Could you check a few things on this model? Use its own coordinates, in mm. A direction names the side the tool comes from. Coordinates: 2 decimals unless noted, no trailing zeros. Loops run counter-clockwise (first coordinate to the right, second up) from the corner with the lowest first, then second, coordinate; pieces in that order, holes last. Notation, with made-up numbers: (-7.75, -32) -> (50.25, -32) arc R27 ccw to (50.25, -13) -> close; hole circle Ø7 at (3, 16.25). An arc over 180 degrees is marked (long way). One line per question, with ' | ' between items.
```python
from build123d import *

# Parameters (mm, degrees)
SKETCH1_W                                            = 90
SKETCH1_H                                            = 30
BOSS_EXTRUDE1_DEPTH                                  = 3
SKETCH3_W                                            = 30
SKETCH3_H                                            = 3
BOSS_EXTRUDE2_DEPTH                                  = 60
RIB5_REACH                                           = 80.861
SKETCH8_WALL_W                                       = 225.516409736
SKETCH8_WALL_H                                       = 30
CUT_EXTRUDE2_REACH                                   = 85.03
SKETCH10_R                                           = 1.1
SKETCH12_R                                           = 2.5
CUT_EXTRUDE3_DEPTH                                   = 27
FILLET1_R                                            = 3
CUT_EXTRUDE4_REACH                                   = 85.03
FILLET2_R                                            = 2
CSK_FOR_M2_5_COUNTERSUNK_FLAT_HEAD_SCREW_D           = 2.7
CSK_FOR_M2_5_COUNTERSUNK_FLAT_HEAD_SCREW_CSINK_D     = 5.5
CSK_FOR_M2_5_COUNTERSUNK_FLAT_HEAD_SCREW_CSINK_ANGLE = 90
MIRROR1_AT_THE_SECOND_PLANE_COPY_1_D                 = 2.7
MIRROR1_AT_THE_SECOND_PLANE_COPY_1_CSINK_D           = 5.5
MIRROR1_AT_THE_SECOND_PLANE_COPY_1_CSINK_ANGLE       = 90


with BuildPart() as part:
    # Sketch1 → Boss-Extrude1 (new body)
    with BuildSketch(Plane(origin=(0, 0, 0), x_dir=(1, 0, 0), z_dir=(0, 1, 0))):
        Rectangle(SKETCH1_W, SKETCH1_H)
    extrude(amount=BOSS_EXTRUDE1_DEPTH)

    # Sketch3 → Boss-Extrude2 (add)
    with BuildSketch(Plane(origin=(0, 3, 0), x_dir=(1, 0, 0), z_dir=(0, 1, 0))):
        with Locations((0, -13.5)):
            Rectangle(SKETCH3_W, SKETCH3_H)
    extrude(amount=BOSS_EXTRUDE2_DEPTH)

    # Sketch8 wall → Rib5 (add, up to next)
    with BuildSketch(Plane(origin=(0, 33, -1.5), x_dir=(0, -0.911921505175, -0.410364677329), z_dir=(0, 0.410364677329, -0.911921505175)), mode=Mode.PRIVATE) as rib5_sk1:
        Rectangle(SKETCH8_WALL_W, SKETCH8_WALL_H)
    rib5_tool1 = extrude(rib5_sk1.sketch, amount=-RIB5_REACH, mode=Mode.PRIVATE) - part.part
    add(rib5_tool1.solids().sort_by_distance((0, 33, -1.5))[0])

    # Cut-Extrude2: up to this plane
    cut_extrude2_end = Plane(origin=(0, 63, 12), z_dir=(0, -0.410364677328798, 0.9119215051751063))
    # Sketch10 → Cut-Extrude2 (cut, up to the surface)
    with BuildSketch(Plane.XY.offset(15), mode=Mode.PRIVATE) as cut_extrude2_sk1:
        with Locations((-10, 56.3)):
            Circle(SKETCH10_R)
    cut_extrude2_tool1 = split(extrude(cut_extrude2_sk1.sketch, amount=-CUT_EXTRUDE2_REACH, mode=Mode.PRIVATE), bisect_by=cut_extrude2_end, keep=Keep.BOTH, mode=Mode.PRIVATE)
    add(cut_extrude2_tool1.solids().sort_by_distance((-10, 56.3, 15))[0], mode=Mode.SUBTRACT)
    # Sketch10 → Cut-Extrude2 (cut, up to the surface)
    with BuildSketch(Plane.XY.offset(15), mode=Mode.PRIVATE) as cut_extrude2_sk2:
        with Locations(Location((10, 56.3, 0), (0, 0, 90))):
            Circle(SKETCH10_R)
    cut_extrude2_tool2 = split(extrude(cut_extrude2_sk2.sketch, amount=-CUT_EXTRUDE2_REACH, mode=Mode.PRIVATE), bisect_by=cut_extrude2_end, keep=Keep.BOTH, mode=Mode.PRIVATE)
    add(cut_extrude2_tool2.solids().sort_by_distance((10, 56.3, 15))[0], mode=Mode.SUBTRACT)
    # Sketch10 → Cut-Extrude2 (cut, up to the surface)
    with BuildSketch(Plane.XY.offset(15), mode=Mode.PRIVATE) as cut_extrude2_sk3:
        with Locations((10, 9.7)):
            Circle(SKETCH10_R)
    cut_extrude2_tool3 = split(extrude(cut_extrude2_sk3.sketch, amount=-CUT_EXTRUDE2_REACH, mode=Mode.PRIVATE), bisect_by=cut_extrude2_end, keep=Keep.BOTH, mode=Mode.PRIVATE)
    add(cut_extrude2_tool3.solids().sort_by_distance((10, 9.7, 15))[0], mode=Mode.SUBTRACT)
    # Sketch10 → Cut-Extrude2 (cut, up to the surface)
    with BuildSketch(Plane.XY.offset(15), mode=Mode.PRIVATE) as cut_extrude2_sk4:
        with Locations(Location((-10, 9.7, 0), (0, 0, 90))):
            Circle(SKETCH10_R)
    cut_extrude2_tool4 = split(extrude(cut_extrude2_sk4.sketch, amount=-CUT_EXTRUDE2_REACH, mode=Mode.PRIVATE), bisect_by=cut_extrude2_end, keep=Keep.BOTH, mode=Mode.PRIVATE)
    add(cut_extrude2_tool4.solids().sort_by_distance((-10, 9.7, 15))[0], mode=Mode.SUBTRACT)

    # Sketch12 → Cut-Extrude3 (cut)
    with BuildSketch(Plane(origin=(0, 0, -15), x_dir=(-1, 0, 0), z_dir=(0, 0, -1))):
        with Locations((-10, 56.3)):
            Circle(SKETCH12_R)
        with Locations((10, 56.3)):
            Circle(SKETCH12_R)
        with Locations((10, 9.7)):
            Circle(SKETCH12_R)
        with Locations((-10, 9.7)):
            Circle(SKETCH12_R)
    extrude(amount=-CUT_EXTRUDE3_DEPTH, mode=Mode.SUBTRACT)

    # Fillet1
    fillet1_edges = [part.edges().sort_by_distance(p)[0] for p in [
        (-45, 1.5, -15),
        (45, 1.5, -15),
    ]]
    fillet(fillet1_edges, radius=FILLET1_R)

    # Cut-Extrude4: up to this plane
    cut_extrude4_end = Plane(origin=(0, 63, 12), z_dir=(0, -0.410364677328798, 0.9119215051751063))
    # Sketch13 → Cut-Extrude4 (cut, up to the surface)
    with BuildSketch(Plane.XY.offset(15), mode=Mode.PRIVATE) as cut_extrude4_sk1:
        Polygon((0, 20), (-13, 33), (0, 46), (13, 33), align=None)
    cut_extrude4_tool1 = split(extrude(cut_extrude4_sk1.sketch, amount=-CUT_EXTRUDE4_REACH, mode=Mode.PRIVATE), bisect_by=cut_extrude4_end, keep=Keep.BOTH, mode=Mode.PRIVATE)
    add(cut_extrude4_tool1.solids().sort_by_distance((0, 33, 15))[0], mode=Mode.SUBTRACT)

    # Fillet2
    fillet2_edges = [part.edges().sort_by_distance(p)[0] for p in [
        (13, 33, 6.75),
        (0, 20, 3.825),
        (-13, 33, 6.75),
        (0, 46, 9.675),
    ]]
    fillet(fillet2_edges, radius=FILLET2_R)

    # CSK for M2.5 Countersunk Flat Head Screw2 (through all)
    with Locations(Plane(origin=(-23, 0, 9), x_dir=(0, 0, -1), z_dir=(0, -1, 0))):
        with Locations((0, 0), (0, -14)):
            csk_for_m2_5_countersunk_flat_head_screw = CounterSinkHole(CSK_FOR_M2_5_COUNTERSUNK_FLAT_HEAD_SCREW_D / 2, CSK_FOR_M2_5_COUNTERSUNK_FLAT_HEAD_SCREW_CSINK_D / 2, counter_sink_angle=CSK_FOR_M2_5_COUNTERSUNK_FLAT_HEAD_SCREW_CSINK_ANGLE)

    # Mirror1: CSK for M2.5 Countersunk Flat Head Screw2 across plane
    add(csk_for_m2_5_countersunk_flat_head_screw.mirror(Plane(origin=(0, 0, 0), x_dir=(0, 0, 1), z_dir=(1, 0, 0))), mode=Mode.SUBTRACT)

    # Mirror1 at the second plane: CSK for M2.5 Countersunk Flat Head Screw2 across plane
    add(csk_for_m2_5_countersunk_flat_head_screw.mirror(Plane.XY), mode=Mode.SUBTRACT)

    # Mirror1 at the second plane copy 1 (through all)
    with Locations(Plane(origin=(23, 0, -9), x_dir=(0, 0, 1), z_dir=(0, -1, 0))):
        with Locations((0, 0), (0, -14)):
            CounterSinkHole(MIRROR1_AT_THE_SECOND_PLANE_COPY_1_D / 2, MIRROR1_AT_THE_SECOND_PLANE_COPY_1_CSINK_D / 2, counter_sink_angle=MIRROR1_AT_THE_SECOND_PLANE_COPY_1_CSINK_ANGLE)


solid = part.part
```
Q1. We'd pull the mould along Y, two halves only. Please class faces 4 (the face through (-45, 1, 2)), 5 (the face through (-30, 3, 0)), 6 (the face through (0.02, 20.83, 3.8)): released by +Y, released by -Y, zero draft, split by the parting line, or undercut.
Values follow:
face 4: zero draft | face 5: released by +Y | face 6: undercut
Q2. Imagine slicing it at A-A on x = -10. Write out the boundary of the cut face in (y, z).
Values follow:
outline: (0, -15) -> (3, -15) -> (7.2, -13.11) -> (7.2, 12) -> (8.6, 12) -> (8.6, 15) -> (0, 15) -> close; (10.8, 12) -> (12.2, 12) -> (12.2, -10.86) -> (30, -2.85) -> (30, 15) -> (10.8, 15) -> close; (36, -0.15) -> (53.8, 7.86) -> (53.8, 12) -> (55.2, 12) -> (55.2, 15) -> (36, 15) -> close; (57.4, 12) -> (58.8, 12) -> (58.8, 10.11) -> (63, 12) -> (63, 15) -> (57.4, 15) -> close
Q3. Please list where these lines run through material, in increasing order: L1, parallel to X at y = 2.15, z = 9; L2, parallel to X at y = 9.7, z = 2.25; L3, parallel to Y at x = 10, z = 12.95. Write a range as [from, to].
Values follow:
L1: x = [-45, -38.35], [-35.65, -24.35], [-21.65, 21.65], [24.35, 35.65], [38.35, 45] | L2: x = [-15, -12.5], [-7.5, 7.5], [12.5, 15] | L3: y = [0, 8.6], [10.8, 30], [36, 55.2], [57.4, 63]
Q4. Imagine slicing it at B-B on z = -9. Give the number of separate pieces and of enclosed holes in the cut face, plus the area to 3 significant figures.
Values follow:
separate pieces: 5 | enclosed holes: 2 | area: 590 mm2
Q5. For pin 1 (9 mm diameter, centred on y = 23, z = -0.5, fed in from +X); pin 2 (1.6 mm diameter, centred on x = -23, z = -9, fed in from -Y); pin 3 (1.5 mm diameter, centred on y = 19.5, z = -3.5, fed in from -X); pin 4 (3 mm diameter, centred on x = 27.5, z = 8, fed in from +Y), each with a flat end and sliding along its axis, tell me the tip position at first contact or that it passes through.
Values follow:
pin 1: stops at x = 15 | pin 2: passes through | pin 3: stops at x = -15 | pin 4: stops at y = 3
Q6. Imagine slicing it at C-C on x = 23. Write out the boundary of the cut face in (y, z), plus the area to 3 significant figures.
Values follow:
outline: (0, -15) -> (3, -15) -> (3, -10.35) -> (1.4, -10.35) -> (0, -11.75) -> close; (0, -6.25) -> (1.4, -7.65) -> (3, -7.65) -> (3, 7.65) -> (1.4, 7.65) -> (0, 6.25) -> close; (0, 11.75) -> (1.4, 10.35) -> (3, 10.35) -> (3, 15) -> (0, 15) -> close | area: 69.9 mm2
Q7. Imagine slicing it at D-D on z = 0.5. Write out the boundary of the cut face in (x, y).
Values follow:
outline: (-45, 0) -> (45, 0) -> (45, 3) -> (15, 3) -> (15, 37.44) -> (8.56, 37.44) -> (11.59, 34.41) arc R2 cw to (11.59, 31.59) -> (1.41, 21.41) arc R2 cw to (-1.41, 21.41) -> (-11.59, 31.59) arc R2 cw to (-11.59, 34.41) -> (-8.56, 37.44) -> (-15, 37.44) -> (-15, 3) -> (-45, 3) -> close; hole circle Ø5 at (-10, 9.7); hole circle Ø5 at (10, 9.7)
Q8. For faces 1 (the face through (15, 23, 5)), 2 (the face through (-6, 26, 4)), 3 (the face through (-11, 55, 12)), which set-ups out of +Z, -Z, +X, -X, +Y, -Y let a thin tool reach every point of the face, with its end or its side?
Values follow:
face 1: +Z, -Z, +X, +Y | face 2: +Z, -Z | face 3: -Z
